```python
from build123d import *

# Parameters (mm, degrees)
BOSS_EXTRUDE1_DEPTH = 250
SKETCH2_R           = 2
CUT_EXTRUDE1_DEPTH  = 1
SKETCH3_W           = 15
SKETCH3_H           = 6
CUT_EXTRUDE2_DEPTH  = 1


with BuildPart() as part:
    # Sketch1 → Boss-Extrude1 (new body)
    with BuildSketch(Plane.XY):
        Polygon((0, 0), (25.4, 0), (25.4, 1), (1, 1), (1, 25.4), (0, 25.4), align=None)
    extrude(amount=-BOSS_EXTRUDE1_DEPTH)

    # Sketch2 → Cut-Extrude1 (cut)
    with BuildSketch(Plane(origin=(0, 1, 0), x_dir=(1, 0, 0), z_dir=(0, 1, 0))):
        with Locations(Location((8.4, 8, 0), (0, 0, 180))):
            Circle(SKETCH2_R)
        with Locations(Location((17.4, 8, 0), (0, 0, 180))):
            Circle(SKETCH2_R)
        with Locations(Location((8.4, 242, 0), (0, 0, 180))):
            Circle(SKETCH2_R)
        with Locations(Location((17.4, 242, 0), (0, 0, 180))):
            Circle(SKETCH2_R)
    extrude(amount=-CUT_EXTRUDE1_DEPTH, mode=Mode.SUBTRACT)

    # Sketch3 → Cut-Extrude2 (cut)
    with BuildSketch(Plane(origin=(1, 0, 0), x_dir=(0, 0, -1), z_dir=(1, 0, 0))):
        with Locations((57.5, 22.4)):
            Rectangle(SKETCH3_W, SKETCH3_H)
    extrude(amount=-CUT_EXTRUDE2_DEPTH, mode=Mode.SUBTRACT)


solid = part.part
```
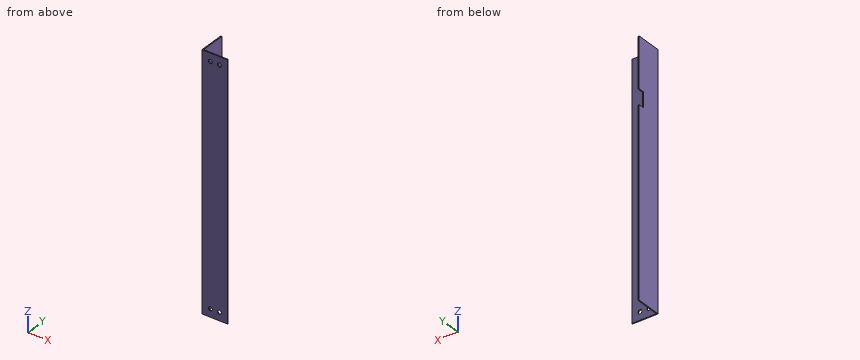
Could you check a few things on this model? Use its own coordinates, in mm. Round coordinates to 2 decimals unless told otherwise and drop trailing zeros. Loops run counter-clockwise (first coordinate to the right, second up) from the corner with the lowest first, then second, coordinate; pieces in that order, holes last. Notation, with made-up numbers: M 38,-37.5 L 60,-37.5 A30 cw 60,-7.5 Z; hole C 85,-35.75 d1. An arc over 180 degrees is marked long. Answer as CSV lines item,"result".
1) Imagine slicing it at A-A on y = 23.25. List the corners of the cut face in (x, z) for me.
From the geometry:
outline,"M 0,-250 L 1,-250 L 1,-65 L 0,-65 Z; M 0,-50 L 1,-50 L 1,0 L 0,0 Z"
2) If I drill on probe 1 along X at (y, z) = (0.3, -242); probe 2 along Z at (x, y) = (8.4, 0.3); probe 3 along X at (y, z) = (5.25, -205.5), over which ranges is the centre line in solid material (lowest first)?
From the geometry:
probe 1,"0 to 6.4, 10.4 to 15.4, 19.4 to 25.4"
probe 2,"-250 to -244, -240 to -10, -6 to 0"
probe 3,"0 to 1"
3) For pin 1 Ø1.5 at (y, z) = (5.5, -183) entering from +X; pin 2 Ø3 at (x, z) = (13, -66.5) entering from +Y; pin 3 Ø0.8 at (x, z) = (0.5, -57.5) entering from +Y; pin 4 Ø3 at (x, z) = (17.4, -8) entering from +Y, each with a flat end and sliding along its axis, tell me the tip position at first contact or that it passes through.
From the geometry:
pin 1,"x = 1"
pin 2,"y = 1"
pin 3,"y = 19.4"
pin 4,"through"
4) Imagine slicing it at C-C on y = 13.25. List the corners of the cut face in (x, z) for me.
From the geometry:
outline,"M 0,-250 L 1,-250 L 1,0 L 0,0 Z"
5) Imagine slicing it at B-B on z = -175.5. List the corners of the cut face in (x, y) for me.
From the geometry:
outline,"M 0,0 L 25.4,0 L 25.4,1 L 1,1 L 1,25.4 L 0,25.4 Z"
